from build123d import *

# Parameters (mm, degrees)
SKETCH2_W           = 350
SKETCH2_H           = 350
SKETCH2_R           = 1.8
SKETCH2_R_2         = 1.5
SKETCH2_W_2         = 12.9979177
SKETCH2_H_2         = 12.99791772
BOSS_EXTRUDE2_DEPTH = 15


with BuildPart() as part:
    # Sketch2 → Boss-Extrude2 (new body)
    with BuildSketch(Plane(origin=(0, 0, 0), x_dir=(0, 0, -1), z_dir=(1, 0, 0))):
        with Locations((-161.173220858, -113.174460432)):
            Rectangle(SKETCH2_W, SKETCH2_H)
        with Locations((-301.173220858, 26.825539568)):
            Circle(SKETCH2_R, mode=Mode.SUBTRACT)
        with Locations((-301.173220858, -3.174460432)):
            Circle(SKETCH2_R, mode=Mode.SUBTRACT)
        with Locations((-325.173220858, -3.174460432)):
            Circle(SKETCH2_R, mode=Mode.SUBTRACT)
        with Locations((-325.173220858, 26.825539568)):
            Circle(SKETCH2_R, mode=Mode.SUBTRACT)
        with Locations((-301.173220858, -223.174460432)):
            Circle(SKETCH2_R, mode=Mode.SUBTRACT)
        with Locations((-325.173220858, -223.174460432)):
            Circle(SKETCH2_R, mode=Mode.SUBTRACT)
        with Locations((-301.173220858, -253.174460432)):
            Circle(SKETCH2_R, mode=Mode.SUBTRACT)
        with Locations((-325.173220858, -253.174460432)):
            Circle(SKETCH2_R, mode=Mode.SUBTRACT)
        with Locations((-21.173220858, -3.174460432)):
            Circle(SKETCH2_R, mode=Mode.SUBTRACT)
        with Locations((2.826779142, -3.174460432)):
            Circle(SKETCH2_R, mode=Mode.SUBTRACT)
        with Locations((2.826779142, 26.825539568)):
            Circle(SKETCH2_R, mode=Mode.SUBTRACT)
        with Locations((-21.173220858, 26.825539568)):
            Circle(SKETCH2_R, mode=Mode.SUBTRACT)
        with Locations((2.826779142, -223.174460432)):
            Circle(SKETCH2_R, mode=Mode.SUBTRACT)
        with Locations((-21.173220858, -223.174460432)):
            Circle(SKETCH2_R, mode=Mode.SUBTRACT)
        with Locations((-21.173220858, -253.174460432)):
            Circle(SKETCH2_R, mode=Mode.SUBTRACT)
        with Locations((2.826779142, -253.174460432)):
            Circle(SKETCH2_R, mode=Mode.SUBTRACT)
        with Locations((-3.673220858, -263.174460432)):
            Circle(SKETCH2_R_2, mode=Mode.SUBTRACT)
        with Locations((4.98703318, -278.174460432)):
            Circle(SKETCH2_R_2, mode=Mode.SUBTRACT)
        with Locations((-12.333474896, -278.174460432)):
            Circle(SKETCH2_R_2, mode=Mode.SUBTRACT)
        with Locations((-12.333474896, 51.825539568)):
            Circle(SKETCH2_R_2, mode=Mode.SUBTRACT)
        with Locations((4.98703318, 51.825539568)):
            Circle(SKETCH2_R_2, mode=Mode.SUBTRACT)
        with Locations((-3.673220858, 36.825539568)):
            Circle(SKETCH2_R_2, mode=Mode.SUBTRACT)
        with Locations((-318.673220858, 36.825539568)):
            Circle(SKETCH2_R_2, mode=Mode.SUBTRACT)
        with Locations((-327.333474896, 51.825539568)):
            Circle(SKETCH2_R_2, mode=Mode.SUBTRACT)
        with Locations((-310.01296682, 51.825539568)):
            Circle(SKETCH2_R_2, mode=Mode.SUBTRACT)
        with Locations((-327.333474896, -278.174460432)):
            Circle(SKETCH2_R_2, mode=Mode.SUBTRACT)
        with Locations((-310.01296682, -278.174460432)):
            Circle(SKETCH2_R_2, mode=Mode.SUBTRACT)
        with Locations((-318.673220858, -263.174460432)):
            Circle(SKETCH2_R_2, mode=Mode.SUBTRACT)
        Polygon((-161.173220858, -38.174460432), (-136.173220858, -38.174460432), (-136.173220858, -45.674460432), (-186.173220858, -45.674460432), (-186.173220858, -38.174460432), align=None, mode=Mode.SUBTRACT)
        with Locations((-60.973061718, 11.825539568)):
            Rectangle(SKETCH2_W_2, SKETCH2_H_2, mode=Mode.SUBTRACT)
        with Locations((-261.373379998, 11.825539568)):
            Rectangle(SKETCH2_W_2, SKETCH2_H_2, mode=Mode.SUBTRACT)
        with Locations((-60.973061718, -238.174460432)):
            Rectangle(SKETCH2_W_2, SKETCH2_H_2, mode=Mode.SUBTRACT)
        with Locations((-261.373379998, -238.174460432)):
            Rectangle(SKETCH2_W_2, SKETCH2_H_2, mode=Mode.SUBTRACT)
        Polygon((-161.173220858, -105.174460432), (-136.173220858, -105.174460432), (-136.173220858, -97.674460432), (-186.173220858, -97.674460432), (-186.173220858, -105.174460432), align=None, mode=Mode.SUBTRACT)
    extrude(amount=BOSS_EXTRUDE2_DEPTH)


solid = part.part
Geometry: final body of the model. Coordinates: model frame, mm. A direction names the side the tool comes from. Give positions to 0.01 mm unless a question says otherwise; leave off trailing zeros. Write each loop counter-clockwise with the first axis right and the second up, starting at its lowest first coordinate (ties: lowest second). Pieces come first, ordered by that corner, then holes. Notation, with made-up numbers: (-14, -16.5) - (5, -16.5) arc R29 cw to (5, 9.5) - close; hole circle Ø10 at (-16, 47.25). An arc over 180 degrees is marked (long way). Return JSON: item names as keys, results as strings. Group by question number.
1) Line query: line 1 (Y direction, x = 13, z = 147.5); line 2 (Z direction, x = 1.75, y = -243); line 3 (Y direction, x = 5.75, z = 260). Output: solid intervals per line, ascending.
2) Set-up query: faces 5 (the flat face through (7, -288.174, 164)), 6 (the flat face through (7, -231.676, 261)). Return all of +Z, -Z, +X, -X, +Y, -Y with unobstructed straight access to the full face (end or side cutting, diameter ignored); none if empty.
3) Mould query, pull axis Z, two halves, no side actions, for faces 1 (the flat face through (7, -38.174, 162)), 2 (the flat face through (0, -111, 164)), 3 (the flat face through (7, -116, -13.827)), 4 (the flat face through (7, -238, 54.474)). Classes: released by +Z, released by -Z, zero draft, split by the parting line, or undercut.
4) Section B-B on y = -238. Return the cut outline in (x, z).
5) Section A-A on z = 259.5. Return the cut outline in (x, y).
Filled in:
{
 "1": {"line 1": "y = -288.17 to -105.17, -97.67 to -45.67, -38.17 to 61.83", "line 2": "z = -13.83 to 54.47, 67.47 to 254.87, 267.87 to 336.17", "line 3": "y = -288.17 to -244.67, -231.68 to 5.33, 18.32 to 61.83"},
 "2": {"face 5": "+Z, -Z, +X, -X, -Y", "face 6": "+X, -X"},
 "3": {"face 1": "undercut", "face 2": "zero draft", "face 3": "released by -Z", "face 4": "undercut"},
 "4": {"outline": "(0, -13.83) - (15, -13.83) - (15, 54.47) - (0, 54.47) - close; (0, 67.47) - (15, 67.47) - (15, 254.87) - (0, 254.87) - close; (0, 267.87) - (15, 267.87) - (15, 336.17) - (0, 336.17) - close"},
 "5": {"outline": "(0, -288.17) - (15, -288.17) - (15, -244.67) - (0, -244.67) - close; (0, -231.68) - (15, -231.68) - (15, 5.33) - (0, 5.33) - close; (0, 18.32) - (15, 18.32) - (15, 61.83) - (0, 61.83) - close"}
}
